The drawing under review shows one solid part. Ordinate dimensions are in mm from its lowest x, y, z. Coordinates: 2 decimals unless noted, no trailing zeros. Write each loop counter-clockwise with the first axis right and the second up, starting at its lowest first coordinate (ties: lowest second). Pieces come first, ordered by that corner, then holes.
Q1. For probe 1 along Z at (x, y) = (172, 1.6); probe 2 along Z at (x, y) = (123, 0.9), list the stretches that pass through material, from the lowest coordinate up.
Q2. Insertion check: pin 1 (2.5 mm diameter, centred on x = 8, z = 8, fed in from -Y) (3 decimals). The pin has a flat end and moves straight along its axis. Give the tip position at first contact, or say it passes through.
Q3. Take a section at A-A (x = 119). Give the boundary of the cut face in (y, z).
Q4. Take a section at B-B (y = 2.2). State how many separate pieces and enclosed holes the cut face has, and give its area (3 significant figures).
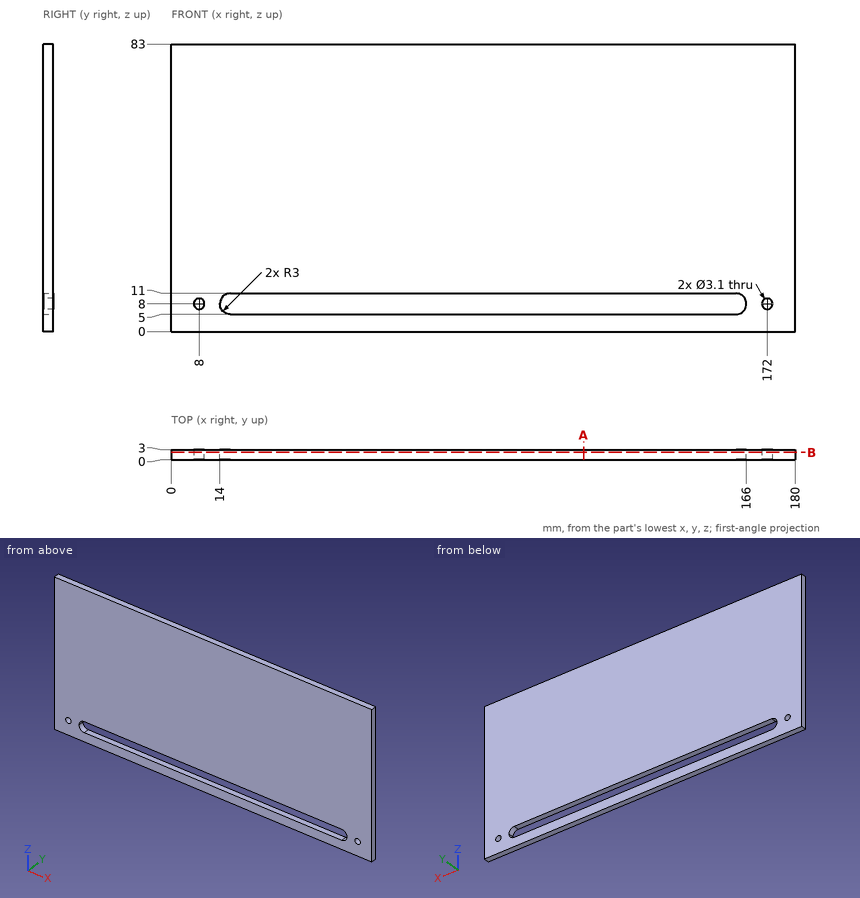
Response:
1. probe 1: z = 0 to 6.45, 9.55 to 83
1. probe 2: z = 0 to 5, 11 to 83
2. pin 1: passes through
3. outline: (0, 0) - (3, 0) - (3, 5) - (0, 5) - close; (0, 11) - (3, 11) - (3, 83) - (0, 83) - close
4. separate pieces: 1
4. enclosed holes: 3
4. area: 14,000 mm2
